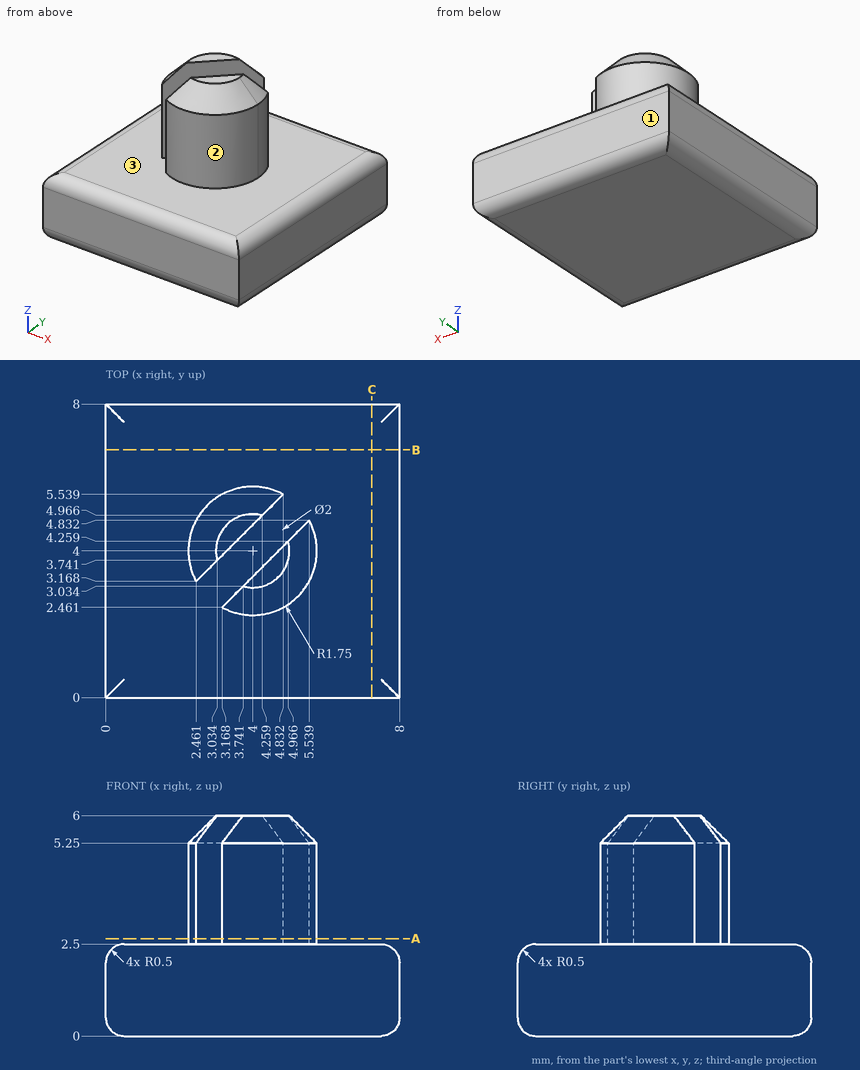
Drawing for the job (mm, zero at the part's lowest x, y, z). A direction names the side the tool comes from. Round coordinates to 2 decimals unless told otherwise and drop trailing zeros. Write each loop counter-clockwise with the first axis right and the second up, starting at its lowest first coordinate (ties: lowest second). Pieces come first, ordered by that corner, then holes.
Item 1: Tool access for the marked faces 1, 2 and 3: list every direction of +Z, -Z, +X, -X, +Y, -Y with a clear straight run to the whole face (end or side of a thin tool).
Filled in:
face 1: +Z, -Z, +X, -X, +Y
face 2: +Z, -Y
face 3: +Z
Item 2: Drop flat-ended pins along their axis: pin 1 Ø1.5 at (x, z) = (4.5, 5) entering from -Y; pin 2 Ø2 at (y, z) = (4, 4) entering from -X. Give the stop position or say it passes through.
Filled in:
pin 1: stops at y = 2.25
pin 2: stops at x = 2.25
Item 3: Band-saw the part on B-B on y = 6.75. Write the cut outline in (x, z).
Filled in:
outline: (0, 0.5) arc R0.5 ccw to (0.5, 0) - (7.5, 0) arc R0.5 ccw to (8, 0.5) - (8, 2) arc R0.5 ccw to (7.5, 2.5) - (0.5, 2.5) arc R0.5 ccw to (0, 2) - close
Item 4: Drill centre lines: L1, parallel to Z at x = 4.75, y = 5.75; L2, parallel to X at y = 6.25, z = 2.25; L3, parallel to Z at x = 4.25, y = 2.5. Where is each one in solid material? Low to high.
Filled in:
L1: z = 0 to 2.5
L2: x = 0.07 to 7.93
L3: z = 0 to 5.48
Item 5: Band-saw the part on A-A on z = 2.65. Write the cut outline in (x, y).
Filled in:
outline: (2.46, 3.17) - (4.83, 5.54) arc R1.75 ccw to start; (3.17, 2.46) arc R1.75 ccw to (5.75, 4) arc R1.75 ccw to (5.54, 4.83) - close
